Source: CAD feature listing. Evaluate the final solid. Frame: model axes, mm. Face numbers are marked on the shaded views. Round coordinates to 2 decimals unless told otherwise and drop trailing zeros. Write each loop counter-clockwise with the first axis right and the second up, starting at its lowest first coordinate (ties: lowest second). Pieces come first, ordered by that corner, then holes.
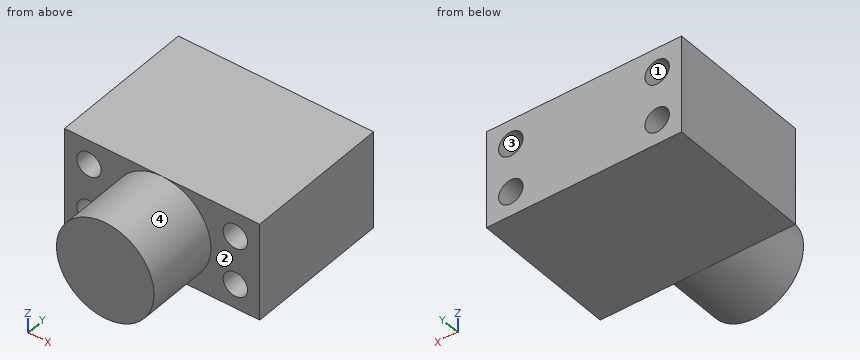
```python
from build123d import *

# Parameters (mm, degrees)
F0_W     = 101.6
F0_H     = 50.8
F1_DEPTH = 76.2
F2_R     = 6.35
F3_DEPTH = 76.201
F4_W     = 25.4
F4_H     = 38.1


with BuildPart() as f1:
    # F0 (on Front) → F1 (new body)
    with BuildSketch(Plane.XZ):
        Rectangle(F0_W, F0_H)
    extrude(amount=F1_DEPTH)

    # F2 (on face) → F3 (cut, through all)
    with BuildSketch(Plane.XZ.offset(76.2)):
        with Locations((-38.1, 12.7)):
            Circle(F2_R)
        with Locations((-38.1, -12.7)):
            Circle(F2_R)
        with Locations((38.1, 12.7)):
            Circle(F2_R)
        with Locations((38.1, -12.7)):
            Circle(F2_R)
    extrude(amount=-F3_DEPTH, mode=Mode.SUBTRACT)

    # F4 (on Top) → F5 (revolve)
    with BuildSketch(Plane.XY):
        with Locations((-12.7, -95.25)):
            Rectangle(F4_W, F4_H)
    revolve(axis=Axis((0, -95.25, 0), (0, -1, 0)))


solid = f1.part
```
Q1. Section query D-D, the plane z = -10. Output: boundary loops of the cut face in (x, y), and give its area (3 significant figures).
Q2. Pin query (flat end, axial travel): P1, Ø1, axis at x = 18, y = -91.5, coming from the -Z side; P2, Ø16.5, axis at x = 38.1, z = -12.7, coming from the -Y side; P3, Ø1.5, axis at x = 21.5, y = -81, coming from the -Z side; P4, Ø10, axis at x = -38.1, z = -12.7, coming from the -Y side. Return the tip coordinate at first contact, or that it passes through.
Q3. Section query B-B, the plane y = -48.5. Output: boundary loops of the cut face in (x, z).
Q4. Mould query, pull axis Z, two halves, no side actions, for the marked faces 1, 2, 3 and 4. Classes: pulls with the +Z half, pulls with the -Z half, needs draft (parallel to the pull), parting line crosses it, or undercut.
Q5. Line query: line 1 (Z direction, x = 38.1, y = -19.5); line 2 (X direction, y = -43.5, z = -14); line 3 (X direction, y = -41, z = -10.5). Output: solid intervals per line, ascending.
Q6. Section query A-A, the plane x = 38.1. Output: boundary loops of the cut face in (y, z).
Q7. Section query C-C, the plane z = 0. Output: boundary loops of the cut face in (x, y), and give its area (3 significant figures).
Filled in:
1. outline: (-50.8, -76.2) - (-43.85, -76.2) - (-43.85, 0) - (-50.8, 0) - close; (-32.35, -76.2) - (-23.35, -76.2) - (-23.35, -114.3) - (23.35, -114.3) - (23.35, -76.2) - (32.35, -76.2) - (32.35, 0) - (-32.35, 0) - close; (43.85, -76.2) - (50.8, -76.2) - (50.8, 0) - (43.85, 0) - close
1. area: 7,770 mm2
2. P1: stops at z = -18.41
2. P2: stops at y = -76.2
2. P3: stops at z = -14.65
2. P4: passes through
3. outline: (-50.8, -25.4) - (50.8, -25.4) - (50.8, 25.4) - (-50.8, 25.4) - close; hole circle Ø12.7 at (-38.1, -12.7); hole circle Ø12.7 at (-38.1, 12.7); hole circle Ø12.7 at (38.1, -12.7); hole circle Ø12.7 at (38.1, 12.7)
4. face 1: undercut
4. face 2: needs draft
4. face 3: undercut
4. face 4: parting line crosses it
5. line 1: z = -25.4 to -19.05, -6.35 to 6.35, 19.05 to 25.4
5. line 2: x = -50.8 to -44.32, -31.88 to 31.88, 44.32 to 50.8
5. line 3: x = -50.8 to -44.06, -32.14 to 32.14, 44.06 to 50.8
6. outline: (-76.2, -25.4) - (0, -25.4) - (0, -19.05) - (-76.2, -19.05) - close; (-76.2, -6.35) - (0, -6.35) - (0, 6.35) - (-76.2, 6.35) - close; (-76.2, 19.05) - (0, 19.05) - (0, 25.4) - (-76.2, 25.4) - close
7. outline: (-50.8, -76.2) - (-25.4, -76.2) - (-25.4, -114.3) - (25.4, -114.3) - (25.4, -76.2) - (50.8, -76.2) - (50.8, 0) - (-50.8, 0) - close
7. area: 9,680 mm2
